from build123d import *

# Parameters (mm, degrees)
SKETCH_W        = 53
SKETCH_H        = 37.5
SKETCH_W_2      = 49
SKETCH_H_2      = 33.5
PAD_DEPTH       = 32
SKETCH001_W     = 53
SKETCH001_H     = 37.5
PAD001_DEPTH    = 2
SKETCH002_W     = 53
SKETCH002_H     = 37.5
PAD002_DEPTH    = 2
SKETCH003_W     = 33.5
SKETCH003_H     = 32
POCKET_DEPTH    = 2
SKETCH004_W     = 10
SKETCH004_H     = 5.75
SKETCH004_W_2   = 12.5
POCKET001_DEPTH = 5
SKETCH005_W     = 51
SKETCH005_H     = 1.8
SKETCH005_H_2   = 1.5
PAD003_DEPTH    = 33.5
SKETCH006_W     = 30.5
SKETCH006_H     = 9
POCKET002_DEPTH = 51
SKETCH007_W     = 17.616245
SKETCH007_H     = 6
PAD004_DEPTH    = 5
SKETCH008_R     = 0.8
POCKET003_DEPTH = 5
SKETCH009_W     = 17.616245
SKETCH009_H     = 6
PAD005_DEPTH    = 3.5
SKETCH010_R     = 0.8
POCKET004_DEPTH = 6
CHAMFER_SIZE    = 3.499
CHAMFER001_SIZE = 4.99
FILLET_R        = 1.99
SKETCH011_W     = 53
SKETCH011_H     = 4
PAD006_DEPTH    = 6
FILLET001_R     = 4


with BuildPart() as part:
    # Sketch → Pad (new body)
    with BuildSketch(Plane.XY):
        Rectangle(SKETCH_W, SKETCH_H)
        Rectangle(SKETCH_W_2, SKETCH_H_2, mode=Mode.SUBTRACT)
    extrude(amount=PAD_DEPTH)

    # Sketch001 (on Face10 of Pad) → Pad001 (join)
    with BuildSketch(Plane.XY.offset(32)):
        Rectangle(SKETCH001_W, SKETCH001_H)
    extrude(amount=PAD001_DEPTH)

    # Sketch002 (on Face4 of Pad001) → Pad002 (join)
    with BuildSketch(Plane(origin=(0, 0, 0), x_dir=(1, 0, 0), z_dir=(0, 0, -1))):
        Rectangle(SKETCH002_W, SKETCH002_H)
    extrude(amount=PAD002_DEPTH)

    # Sketch003 (on Face3 of Pad002) → Pocket (cut)
    with BuildSketch(Plane.YZ.offset(26.5)):
        with Locations((0, 16)):
            Rectangle(SKETCH003_W, SKETCH003_H)
    extrude(amount=-POCKET_DEPTH, mode=Mode.SUBTRACT)

    # Sketch004 (on Face13 of Pocket) → Pocket001 (cut)
    with BuildSketch(Plane.XY.offset(34)):
        with Locations((-19.3, -11.875)):
            Rectangle(SKETCH004_W, SKETCH004_H)
        with Locations((-5.4, -11.875)):
            Rectangle(SKETCH004_W_2, SKETCH004_H)
        with Locations((8.55, -11.875)):
            Rectangle(SKETCH004_W, SKETCH004_H)
    extrude(amount=-POCKET001_DEPTH, mode=Mode.SUBTRACT)

    # Sketch005 (on Face36 of Pocket001) → Pad003 (join)
    with BuildSketch(Plane(origin=(0, -16.75, 0), x_dir=(-1, 0, 0), z_dir=(0, 1, 0))):
        with Locations((-1, 22.25)):
            Rectangle(SKETCH005_W, SKETCH005_H)
        with Locations((-1, 26)):
            Rectangle(SKETCH005_W, SKETCH005_H_2)
        with Locations((-1, 18.5)):
            Rectangle(SKETCH005_W, SKETCH005_H_2)
    extrude(amount=PAD003_DEPTH)

    # Sketch006 (on Face11 of Pad003) → Pocket002 (cut)
    with BuildSketch(Plane.YZ.offset(26.5)):
        with Locations((0, 22.25)):
            Rectangle(SKETCH006_W, SKETCH006_H)
    extrude(amount=-POCKET002_DEPTH, mode=Mode.SUBTRACT)

    # Sketch007 (on Face57 of Pocket002) → Pad004 (join)
    with BuildSketch(Plane.XY):
        with Locations((17.6918775, 0)):
            Rectangle(SKETCH007_W, SKETCH007_H)
    extrude(amount=PAD004_DEPTH)

    # Sketch008 (on Face24 of Pad004) → Pocket003 (cut)
    with BuildSketch(Plane.YZ.offset(26.5)):
        with Locations((0, 2.5)):
            Circle(SKETCH008_R)
    extrude(amount=-POCKET003_DEPTH, mode=Mode.SUBTRACT)

    # Sketch009 (on Face65 of Pocket003) → Pad005 (join)
    with BuildSketch(Plane(origin=(0, 0, 32), x_dir=(1, 0, 0), z_dir=(0, 0, -1))):
        with Locations((17.6918775, 0)):
            Rectangle(SKETCH009_W, SKETCH009_H)
    extrude(amount=PAD005_DEPTH)

    # Sketch010 (on Face41 of Pad005) → Pocket004 (cut)
    with BuildSketch(Plane.YZ.offset(26.5)):
        with Locations((0, 30.25)):
            Circle(SKETCH010_R)
    extrude(amount=-POCKET004_DEPTH, mode=Mode.SUBTRACT)

    # Chamfer
    chamfer_edges = [part.edges().sort_by_distance(p)[0] for p in [
        (8.883755, 0, 28.5),
    ]]
    chamfer(chamfer_edges, length=CHAMFER_SIZE)

    # Chamfer001
    chamfer001_edges = [part.edges().sort_by_distance(p)[0] for p in [
        (8.883755, 0, 5),
    ]]
    chamfer(chamfer001_edges, length=CHAMFER001_SIZE)

    # Fillet
    fillet_edges = [part.edges().sort_by_distance(p)[0] for p in [
        (0, -18.75, 34),
        (0, 18.75, 34),
        (0, 18.75, -2),
        (0, -18.75, -2),
    ]]
    fillet(fillet_edges, radius=FILLET_R)

    # Sketch011 (on Face5 of Fillet) → Pad006 (join)
    with BuildSketch(Plane(origin=(0, 0, -2), x_dir=(1, 0, 0), z_dir=(0, 0, -1))):
        with Locations((0, 7.65)):
            Rectangle(SKETCH011_W, SKETCH011_H)
        with Locations((0, -7.65)):
            Rectangle(SKETCH011_W, SKETCH011_H)
    extrude(amount=PAD006_DEPTH)

    # Fillet001
    fillet001_edges = [part.edges().sort_by_distance(p)[0] for p in [
        (0, 9.65, -2),
        (0, -9.65, -2),
    ]]
    fillet(fillet001_edges, radius=FILLET001_R)


solid = part.part
Can you work these out from the model? Positions are in its coordinate system, mm. A direction names the side the tool comes from. Give positions to 0.01 mm unless a question says otherwise; leave off trailing zeros. Order: outer loops, then holes, each group sorted by start corner. A loop starts at its lowest first (then second) coordinate and runs counter-clockwise, first axis right, second up. Notation, with made-up numbers: M 40,22.5 L 88,22.5 A16 ccw 88,47.5 Z; hole C 65,-32.75 d10. An arc over 180 degrees is marked long. Use one line per item in the form item = value. Start each with the question number.
Item 1: If we section it at B-B (z = 30.25): Write out the boundary of the cut face in (x, y), then the cut area to 3 significant figures.
Item 2: We'd pull the mould along X, two halves only. Please class faces 1 (the flat face through (-5, -9, 33)), 2 (the flat face through (1, 15.25, 22)), 3 (the flat face through (26.5, 1, 4)): +X half, -X half, draft (parallel to the pull), parting line (faces both ways), or undercut.
Item 3: For faces 4 (the flat face through (10.61, 0.04, 30.27)), 5 (the flat face through (0.85, -12, 33)), 6 (the flat face through (0, 15, -2)), 7 (the cylindrical face through (0.371, -18.183, 33.402)), 8 (the flat face through (1, 15.25, 18)), which set-ups out of +Z, -Z, +X, -X, +Y, -Y let a thin tool reach every point of the face, with its end or its side?
Item 4: If we section it at C-C (y = 8.5): Write out the boundary of the cut face in (x, z).
Item 5: Will these pins go through, and if not, where does the flat tip stop? pin 1 Ø0.6 at (x, z) = (10, 32.5) entering from -Y; pin 2 Ø6.5 at (x, y) = (17, 1) entering from -Z; pin 3 Ø1.6 at (x, z) = (-9, -7) entering from -Y.
Item 6: If we section it at D-D (z = 2.5): Write out the boundary of the cut face in (x, y), then the cut area to 3 significant figures.
Item 7: If I drill on line 1 along Z through (x, y) = (25.1, 0); line 2 along Z through (x, y) = (-9, 16.5); line 3 along Y through (x, z) = (-14, 23), over which ranges is the centre line in solid material (lowest first)?
Outcome:
q1.outline = M -26.5,-18.75 L 26.5,-18.75 L 26.5,-16.75 L -24.5,-16.75 L -24.5,16.75 L 26.5,16.75 L 26.5,18.75 L -26.5,18.75 Z; M 10.63,-3 L 26.5,-3 L 26.5,-0.8 L 20.5,-0.8 L 20.5,0.8 L 26.5,0.8 L 26.5,3 L 10.63,3 Z
q1.area = 365 mm2
q2.face_1 = undercut
q2.face_2 = draft
q2.face_3 = +X half
q3.face_4 = none
q3.face_5 = +Z
q3.face_6 = -Z, +X, -X, +Y
q3.face_7 = +Z, +X, -X, -Y
q3.face_8 = +X
q4.outline = M -26.5,-8 L 26.5,-8 L 26.5,0 L -24.5,0 L -24.5,32 L 26.5,32 L 26.5,34 L -26.5,34 Z
q5.pin_1 = -18.74
q5.pin_2 = -2
q5.pin_3 = -9.65
q6.outline = M -26.5,-18.75 L 26.5,-18.75 L 26.5,-16.75 L -24.5,-16.75 L -24.5,16.75 L 26.5,16.75 L 26.5,18.75 L -26.5,18.75 Z; M 11.37,-3 L 26.5,-3 L 26.5,-0.8 L 21.5,-0.8 L 21.5,0.8 L 26.5,0.8 L 26.5,3 L 11.37,3 Z
q6.area = 362 mm2
q7.line_1 = -2 to 1.7, 3.3 to 5, 28.5 to 29.45, 31.05 to 34
q7.line_2 = -2 to 0, 17.75 to 19.25, 21.35 to 23.15, 25.25 to 26.75, 32 to 34
q7.line_3 = -18.75 to -15.25, 15.25 to 18.75
